```python
from build123d import *

# Parameters (mm, degrees)
SKETCH_W        = 60
SKETCH_H        = 28
SKETCH_R        = 1.7
SKETCH_R_2      = 10.2
SKETCH_R_3      = 2.9
PAD_DEPTH       = 5
SKETCH001_R     = 4.1
POCKET001_DEPTH = 3.2
SKETCH002_W     = 60
SKETCH002_H     = 28
SKETCH002_R     = 2.8
SKETCH002_R_2   = 4.1
PAD001_DEPTH    = 4
SKETCH003_R     = 11.2
POCKET_DEPTH    = 3
SKETCH004_W     = 10
SKETCH004_H     = 9
PAD002_DEPTH    = 10
SKETCH009_R     = 2.9
POCKET002_DEPTH = 9


with BuildPart() as part:
    # Sketch → Pad (new body)
    with BuildSketch(Plane.XY):
        Rectangle(SKETCH_W, SKETCH_H)
        with Locations((10, 8)):
            Circle(SKETCH_R, mode=Mode.SUBTRACT)
        with Locations((25, 8)):
            Circle(SKETCH_R, mode=Mode.SUBTRACT)
        with Locations((10, -8)):
            Circle(SKETCH_R, mode=Mode.SUBTRACT)
        with Locations((25, -8)):
            Circle(SKETCH_R, mode=Mode.SUBTRACT)
        with Locations((-17.5, 0)):
            Circle(SKETCH_R_2, mode=Mode.SUBTRACT)
        Circle(SKETCH_R_3, mode=Mode.SUBTRACT)
    extrude(amount=PAD_DEPTH)

    # Sketch001 (on Face11 of Pad) → Pocket001 (cut)
    with BuildSketch(Plane(origin=(0, 0, 0), x_dir=(1, 0, 0), z_dir=(0, 0, -1))):
        with Locations((25, 8)):
            Circle(SKETCH001_R)
        with Locations((25, -8)):
            Circle(SKETCH001_R)
        with Locations((10, 8)):
            Circle(SKETCH001_R)
        with Locations((10, -8)):
            Circle(SKETCH001_R)
    extrude(amount=-POCKET001_DEPTH, mode=Mode.SUBTRACT)

    # Sketch002 (on Face4 of Pocket001) → Pad001 (join)
    with BuildSketch(Plane(origin=(0, 0, 0), x_dir=(1, 0, 0), z_dir=(0, 0, -1))):
        Rectangle(SKETCH002_W, SKETCH002_H)
        Circle(SKETCH002_R, mode=Mode.SUBTRACT)
        with Locations((10, 8)):
            Circle(SKETCH002_R_2, mode=Mode.SUBTRACT)
        with Locations((10, -8)):
            Circle(SKETCH002_R_2, mode=Mode.SUBTRACT)
        with Locations((25, 8)):
            Circle(SKETCH002_R_2, mode=Mode.SUBTRACT)
        with Locations((25, -8)):
            Circle(SKETCH002_R_2, mode=Mode.SUBTRACT)
    extrude(amount=PAD001_DEPTH)

    # Sketch003 (on Face9 of Pad001) → Pocket (cut)
    with BuildSketch(Plane(origin=(0, 0, -4), x_dir=(1, 0, 0), z_dir=(0, 0, -1))):
        with Locations((-17.5, 0)):
            Circle(SKETCH003_R)
    extrude(amount=-POCKET_DEPTH, mode=Mode.SUBTRACT)

    # Sketch004 (on Face7 of Pocket) → Pad002 (join)
    with BuildSketch(Plane(origin=(-30, 0, 0), x_dir=(0, -1, 0), z_dir=(-1, 0, 0))):
        with Locations((0, 0.5)):
            Rectangle(SKETCH004_W, SKETCH004_H)
    extrude(amount=PAD002_DEPTH)

    # Sketch009 → Pocket002 (cut)
    with BuildSketch(Plane(origin=(0, 0, -4), x_dir=(1, 0, 0), z_dir=(0, 0, -1))):
        with Locations((-35, 0)):
            Circle(SKETCH009_R)
    extrude(amount=-POCKET002_DEPTH, mode=Mode.SUBTRACT)


solid = part.part
```
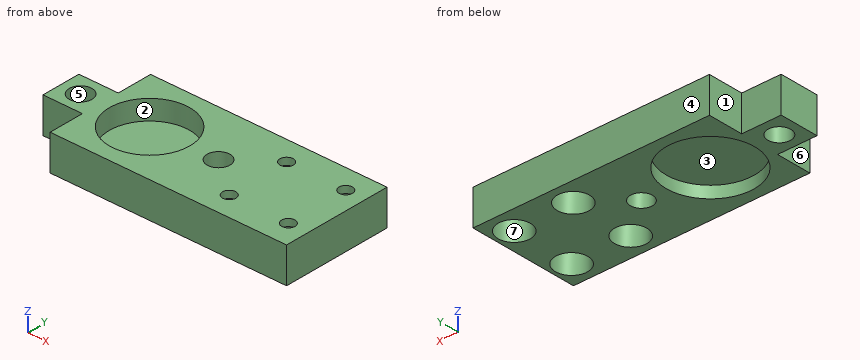
The model under review builds one solid part; all positions refer to its coordinate system, in mm. Face numbers are marked on the shaded views. A direction names the side the tool comes from. Round coordinates to 2 decimals unless told otherwise and drop trailing zeros. Order: outer loops, then holes, each group sorted by start corner. A loop starts at its lowest first (then second) coordinate and runs counter-clockwise, first axis right, second up.
(1) Take a section at A-A, the plane x = 25. State the section outline as (y, z) points.
Working result:
outline: (-14, -4) - (-12.1, -4) - (-12.1, 3.2) - (-9.7, 3.2) - (-9.7, 5) - (-14, 5) - close; (-6.3, 3.2) - (-3.9, 3.2) - (-3.9, -4) - (3.9, -4) - (3.9, 3.2) - (6.3, 3.2) - (6.3, 5) - (-6.3, 5) - close; (9.7, 3.2) - (12.1, 3.2) - (12.1, -4) - (14, -4) - (14, 5) - (9.7, 5) - close
(2) Tool access review of the marked faces 1, 2 and 3: name each direction out of +Z, -Z, +X, -X, +Y, -Y from which nothing blocks a thin tool from reaching the whole face with its end or side.
Working result:
face 1: +Z, -Z, -X, +Y
face 2: +Z
face 3: -Z
(3) Take a section at C-C, the plane x = -35. State the section outline as (y, z) points.
Working result:
outline: (-5, -4) - (-2.9, -4) - (-2.9, 5) - (-5, 5) - close; (2.9, -4) - (5, -4) - (5, 5) - (2.9, 5) - close
(4) Mouldability with a two-part tool opening along X and no side actions: class the marked faces 4, 5, 6 and 7 as released by +X, released by -X, zero draft, split by the parting line, or undercut.
Working result:
face 4: zero draft
face 5: undercut
face 6: released by -X
face 7: undercut
(5) Take a section at D-D, the plane y = 8. State the section outline as (x, z) points, plus the area to 3 significant figures.
Working result:
outline: (-30, -4) - (-25.34, -4) - (-25.34, -1) - (-9.66, -1) - (-9.66, -4) - (5.9, -4) - (5.9, 3.2) - (8.3, 3.2) - (8.3, 5) - (-11.17, 5) - (-11.17, 0) - (-23.83, 0) - (-23.83, 5) - (-30, 5) - close; (11.7, 3.2) - (14.1, 3.2) - (14.1, -4) - (20.9, -4) - (20.9, 3.2) - (23.3, 3.2) - (23.3, 5) - (11.7, 5) - close; (26.7, 3.2) - (29.1, 3.2) - (29.1, -4) - (30, -4) - (30, 5) - (26.7, 5) - close
area: 299 mm2
(6) For P1, Ø4, axis at x = 25, y = -8, coming from the -Z side; P2, Ø1.7, axis at x = -1.5, y = 0, coming from the +Z side (3 decimals); P3, Ø2, axis at y = 7, z = 1, coming from the -X side; P4, Ø4.5, axis at x = -33, z = -0.5, coming from the -Y side, all flat-tipped, find the tip position at first contact; note any pin that passes through.
Working result:
P1: stops at z = 3.2
P2: passes through
P3: stops at x = -30
P4: stops at y = -5
(7) Take a section at B-B, the plane z = 1.5. State the section outline as (x, y) points, plus the area to 3 significant figures.
Working result:
outline: (-40, -5) - (-30, -5) - (-30, -14) - (30, -14) - (30, 14) - (-30, 14) - (-30, 5) - (-40, 5) - close; hole circle Ø5.8 at (-35, 0); hole circle Ø20.4 at (-17.5, 0); hole circle Ø5.8 at (0, 0); hole circle Ø8.2 at (10, -8); hole circle Ø8.2 at (10, 8); hole circle Ø8.2 at (25, -8); hole circle Ø8.2 at (25, 8)
area: 1,190 mm2
(8) Wall thickness on L1, parallel to Y at x = 25, z = 4.25; L2, parallel to Y at x = 25, z = -2.5; L3, parallel to X at y = 0, z = -1.4: over which ranges is each line inside the solid? List them lowest first.
Working result:
L1: y = -14 to -9.7, -6.3 to 6.3, 9.7 to 14
L2: y = -14 to -12.1, -3.9 to 3.9, 12.1 to 14
L3: x = -40 to -37.9, -32.1 to -28.7, -6.3 to -2.8, 2.8 to 30
